from build123d import *

# Parameters (mm, degrees)
F1_DEPTH = 10
F2_R     = 2
F3_DEPTH = 5
F4_R     = 2
F5_DEPTH = 5


with BuildPart() as f1:
    # F0 (on Top) → F1 (new body)
    with BuildSketch(Plane.XY):
        Polygon((0, 20), (0, 0), (20, 0), (20, 4), (17, 4), (15, 3), (7, 3), (5, 5), (3, 7), (3, 15), (4, 17), (4, 20), align=None)
    extrude(amount=F1_DEPTH)

    # F2 (on face) → F3 (cut)
    with BuildSketch(Plane.YZ.offset(3)):
        with Locations((11, 5)):
            Circle(F2_R)
    extrude(amount=-F3_DEPTH, mode=Mode.SUBTRACT)

    # F4 (on face) → F5 (cut)
    with BuildSketch(Plane(origin=(0, 3, 0), x_dir=(-1, 0, 0), z_dir=(0, 1, 0))):
        with Locations((-11, 5)):
            Circle(F4_R)
    extrude(amount=-F5_DEPTH, mode=Mode.SUBTRACT)


solid = f1.part
The listing builds one solid part. Answer for the finished solid, in the listing's coordinates (mm). A direction names the side the tool comes from. Coordinates: 2 decimals unless noted, no trailing zeros. Loops run counter-clockwise (first coordinate to the right, second up) from the corner with the lowest first, then second, coordinate; pieces in that order, holes last. Notation, with made-up numbers: M 88.5,4 L 93.5,4 A20 cw 93.5,19 Z; hole C 89.5,85.5 d7. An arc over 180 degrees is marked long. Answer in a Markdown table with one row per item.
1) Find section A-A (y = 11). Determine the outline of the cut face in (x, z), then the cut area to 3 significant figures.
Answers below:
| item | result |
|---|---|
| outline | M 0,0 L 3,0 L 3,3 L 0,3 Z; M 0,7 L 3,7 L 3,10 L 0,10 Z |
| area | 18.0 mm^2 |
2) Which of the six approach directions +Z, -Z, +X, -X, +Y, -Y give full straight-line access (tool end or side, diameter ignored) to faces 1 (the flat face through (3.5, 16, 4.9)), 2 (the flat face through (16, 3.5, 4.9)), 3 (the flat face through (4, 18, 5))?
Answers below:
| item | result |
|---|---|
| face 1 | +Z, -Z, +X |
| face 2 | +Z, -Z, +Y |
| face 3 | +Z, -Z, +X, +Y |
3) Find section D-D (x = 2.75). Determine the outline of the cut face in (y, z), then the cut area to 3 significant figures.
Answers below:
| item | result |
|---|---|
| outline | M 0,0 L 20,0 L 20,10 L 0,10 Z; hole C 11,5 d4 |
| area | 187 mm^2 |
4) Find section C-C (z = 6.75). Determine the outline of the cut face in (x, y), then the cut area to 3 significant figures.
Answers below:
| item | result |
|---|---|
| outline | M 0,0 L 10.03,0 L 10.03,3 L 7,3 L 3,7 L 3,10.03 L 0,10.03 Z; M 0,11.97 L 3,11.97 L 3,15 L 4,17 L 4,20 L 0,20 Z; M 11.97,0 L 20,0 L 20,4 L 17,4 L 15,3 L 11.97,3 Z |
| area | 115 mm^2 |
5) Determine the mould class of faces 4 (the flat face through (9, 3, 4)), 5 (the flat face through (19, 4, 5)), 6 (the flat face through (0, 8, 5)) for opening direction X: released by +X, released by -X, zero draft, split by the parting line, or undercut.
Answers below:
| item | result |
|---|---|
| face 4 | undercut |
| face 5 | zero draft |
| face 6 | released by -X |
6) Given pin 1 (3.5 mm diameter, centred on x = 18.5, z = 3, fed in from +Y); pin 2 (4 mm diameter, centred on x = 11, z = 4, fed in from +Y); pin 3 (1.5 mm diameter, centred on x = 6.5, y = 5, fed in from -Z); pin 4 (2.5 mm diameter, centred on y = 18, z = 3.5, fed in from +X), each flat-ended and moving along its own axis, determine where each tip first touches the part or whether it passes through.
Answers below:
| item | result |
|---|---|
| pin 1 | y = 4 |
| pin 2 | y = 3 |
| pin 3 | through |
| pin 4 | x = 4 |
7) Find the intervals of material crossed by probe 1 along Z at (x, y) = (11, 0.9); probe 2 along Y at (x, z) = (6, 0.5); probe 3 along Y at (x, z) = (3.75, 1.5), in increasing order.
Answers below:
| item | result |
|---|---|
| probe 1 | 0 to 3, 7 to 10 |
| probe 2 | 0 to 4 |
| probe 3 | 0 to 6.25, 16.5 to 20 |
